Part model, mm, in its own coordinate system. Face numbers are marked on the shaded views. A direction names the side the tool comes from. Coordinates: 2 decimals unless noted, no trailing zeros. Order: outer loops, then holes, each group sorted by start corner. A loop starts at its lowest first (then second) coordinate and runs counter-clockwise, first axis right, second up.
1) Cut at C-C (z = 9.25). Give the number of separate pieces and of enclosed holes in the cut face, and give its area (3 significant figures).
2) Cut at D-D (y = 52.5). List the corners of the cut face in (x, z) (3 decimals).
3) Pin check, flat tips, straight feed: pin 1 Ø1.5 at (x, y) = (7.5, -58) entering from -Z; pin 2 Ø3 at (x, y) = (-8.14, -75.8) entering from -Z; pin 3 Ø2.5 at (y, z) = (0, 4.5) entering from -X; pin 4 Ø3.5 at (y, z) = (-2.5, 4.5) entering from +X. Stop position of each tip, or through.
4) Cut at A-A (x = 0). List the corners of the cut face in (y, z).
5) Cut at B-B (y = 0). List the corners of the cut face in (x, z) (3 decimals), and give its area (3 significant figures).
6) Mould opens along Y. For the marked faces 1, 2, 3 and 4 say: +Y half, -Y half, draft (parallel to the pull), parting line (faces both ways), or undercut.
7) Tool access for the marked faces 5 and 6: list every direction of +Z, -Z, +X, -X, +Y, -Y with a clear straight run to the whole face (end or side of a thin tool).
8) Wall check: L1, parallel to Y at x = 0, z = 9.35; L2, parallel to Y at x = 0, z = 7; L3, parallel to Y at x = 3.25, z = 2.5. Give the ranges that are in metal, low to high.
```python
from build123d import *

# Parameters (mm, degrees)
F0_W      = 24.13
F0_H      = 149.86
F1_DEPTH  = 12.7
F2_W      = 12.446
F2_H      = 20.32
F3_DEPTH  = 0.29765625
F4_R      = 3.96875
F5_DEPTH  = 25.4
F7_R      = 1.7859375
F8_DEPTH  = 25.4
F6_R      = 11.7078125
F9_DEPTH  = 5.159375
F10_R     = 5.3578125
F11_DEPTH = 25.4
F12_R     = 1.7907
F13_DEPTH = 25.4
F14_R     = 5.08
F16_DEPTH = 2.778125


# Not quite as in the source:
# - a length typed as a fraction of an inch, garbled in the dataset ("3 / 203.2 mm" for 3/8 in), is restored


with BuildPart() as f1:
    # F0 (on Top) → F1 (new body)
    with BuildSketch(Plane.XY):
        with Locations((0, -13.97)):
            Rectangle(F0_W, F0_H)
    extrude(amount=F1_DEPTH)

    # F2 (on face) → F3 (cut)
    with BuildSketch(Plane.YZ.offset(12.065)):
        with Locations((0, 2.54)):
            Rectangle(F2_W, F2_H)
    extrude(amount=-F3_DEPTH, mode=Mode.SUBTRACT)

    # F4 (on face) → F5 (cut)
    with BuildSketch(Plane.XY.offset(12.7)):
        with Locations((0, 50.8381508)):
            Circle(F4_R)
    extrude(amount=-F5_DEPTH, mode=Mode.SUBTRACT)

    # F7 (on face) → F8 (cut)
    with BuildSketch(Plane.YZ.offset(11.76734375)):
        with Locations((0, 3.7703125)):
            Circle(F7_R)
    extrude(amount=-F8_DEPTH, mode=Mode.SUBTRACT)

    # F6 (on face) → F9 (cut)
    with BuildSketch(Plane.XY.offset(12.7)):
        with Locations((0, -75.803125)):
            Circle(F6_R)
    extrude(amount=-F9_DEPTH, mode=Mode.SUBTRACT)

    # F10 (on face) → F11 (cut)
    with BuildSketch(Plane.XY.offset(7.540625)):
        with Locations((0, -75.803125)):
            Circle(F10_R)
    extrude(amount=-F11_DEPTH, mode=Mode.SUBTRACT)

    # F12 (on face) → F13 (cut)
    with BuildSketch(Plane.XY.offset(7.540625)):
        with Locations((-8.1359375, -75.803125)):
            Circle(F12_R)
        with Locations((8.1359375, -75.803125)):
            Circle(F12_R)
    extrude(amount=-F13_DEPTH, mode=Mode.SUBTRACT)

    # F14
    f14_edges = [f1.edges().sort_by_distance(p)[0] for p in [
        (-12.065, -88.9, 6.35),
        (12.065, -88.9, 6.35),
        (-12.065, 60.96, 6.35),
        (12.065, 60.96, 6.35),
    ]]
    fillet(f14_edges, radius=F14_R)

    # F15 (on face) → F16 (cut)
    with BuildSketch(Plane(origin=(-12.065, 0, 0), x_dir=(0, -1, 0), z_dir=(-1, 0, 0))):
        Polygon((2.2913588808, 7.7390625), (-2.2913588808, 7.7390625), (-4.5827177617, 3.7703125), (-2.2913588808, -0.1984375), (2.2913588808, -0.1984375), (4.5827177617, 3.7703125), align=None)
    extrude(amount=-F16_DEPTH, mode=Mode.SUBTRACT)


solid = f1.part
```
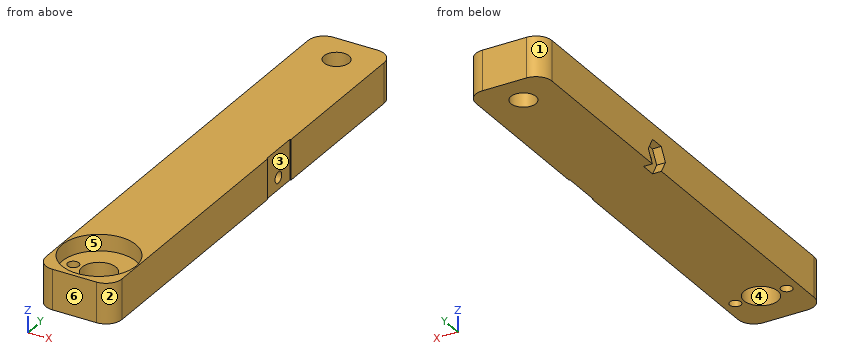
Geometry check:
1. separate pieces: 1
1. enclosed holes: 2
1. area: 3,110 mm2
2. outline: (-12.065, 0) - (-3.604, 0) - (-3.604, 12.7) - (-12.065, 12.7) - close; (3.604, 0) - (12.065, 0) - (12.065, 12.7) - (3.604, 12.7) - close
3. pin 1: stops at z = 0
3. pin 2: passes through
3. pin 3: stops at x = -9.29
3. pin 4: stops at x = 11.77
4. outline: (-88.9, 0) - (-81.16, 0) - (-81.16, 7.54) - (-87.51, 7.54) - (-87.51, 12.7) - (-88.9, 12.7) - close; (-70.45, 0) - (46.87, 0) - (46.87, 12.7) - (-64.1, 12.7) - (-64.1, 7.54) - (-70.45, 7.54) - close; (54.81, 0) - (60.96, 0) - (60.96, 12.7) - (54.81, 12.7) - close; hole circle Ø3.57 at (0, 3.77)
5. outline: (-12.065, 7.739) - (-9.287, 7.739) - (-9.287, 5.556) - (11.767, 5.556) - (11.767, 12.7) - (-12.065, 12.7) - close; (-9.287, 0) - (11.767, 0) - (11.767, 1.984) - (-9.287, 1.984) - close
5. area: 206 mm2
6. face 1: +Y half
6. face 2: -Y half
6. face 3: undercut
6. face 4: undercut
7. face 5: +Z
7. face 6: +Z, -Z, +X, -X, -Y
8. L1: y = -88.9 to -87.51, -64.1 to 46.87, 54.81 to 60.96
8. L2: y = -88.9 to -81.16, -70.45 to 46.87, 54.81 to 60.96
8. L3: y = -88.9 to -80.06, -71.54 to -1.26, 1.26 to 48.56, 53.12 to 60.96
